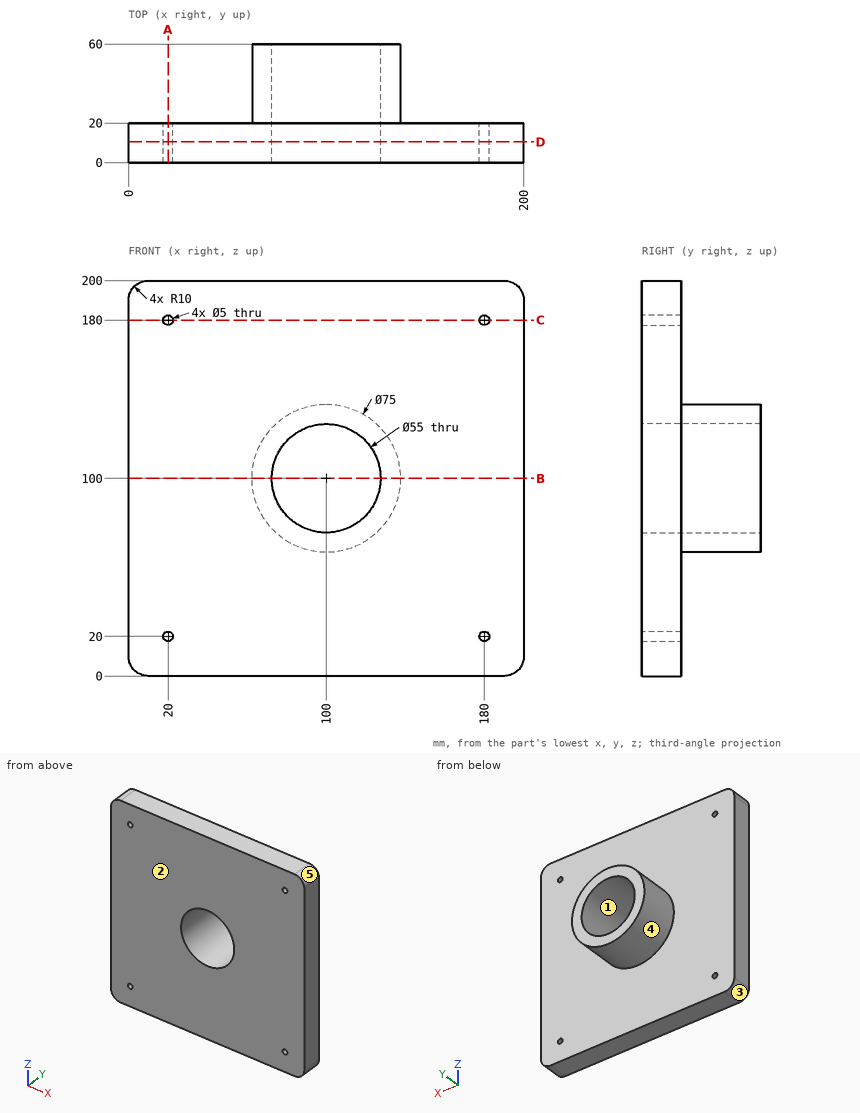
The figure shows three views and two pictorial views of one solid part (mm, origin at its lowest corner). Answer the questions. A direction names the side the tool comes from. Coordinates: 2 decimals unless noted, no trailing zeros. Loops run counter-clockwise (first coordinate to the right, second up) from the corner with the lowest first, then second, coordinate; pieces in that order, holes last. Notation, with made-up numbers: (-35, 66) -> (-5, 66) arc R25 ccw to (-5, 97) -> close; hole circle Ø11 at (-9.5, 19). An arc over 180 degrees is marked (long way). Use one line per item in the form item = value. Start each with the question number.
Item 1: Consider L1, parallel to X at y = 9, z = 180; L2, parallel to Y at x = 101.5, z = 190. Determine where each line is inside the solid, lowest interval first. Write a range as [from, to].
Item 2: Flat-ended cylindrical pins translate along their axes: pin 1 Ø8 at (x, z) = (137, 148) entering from +Y; pin 2 Ø4.5 at (x, z) = (180, 20) entering from +Y. Find the tip coordinate at first contact, or state that the pin passes through.
Item 3: The part is cut by section B-B on z = 100. Determine the outline of the cut face in (x, y), then the cut area to 3 significant figures.
Item 4: The part is cut by section C-C on z = 180. Determine the outline of the cut face in (x, y).
Item 5: The mould has two halves that part along X. Classify the marked faces 1, 2 and 3: released by +X, released by -X, zero draft, split by the parting line, or undercut.
Item 6: The part is cut by section D-D on y = 10.5. Determine the outline of the cut face in (x, z), then the cut area to 3 significant figures.
Item 7: A tool of negligible diameter and unlimited length cuts with its end or side. For the marked faces 4 and 5, from which of +Z, -Z, +X, -X, +Y, -Y can it reach the whole face along a straight path? Write none if from no direction.
Item 8: The part is cut by section A-A on x = 20. Determine the outline of the cut face in (y, z).
Answer key:
q1.L1 = [0, 17.5], [22.5, 177.5], [182.5, 200]
q1.L2 = [0, 20]
q2.pin_1 = 20
q2.pin_2 = through
q3.outline = (0, 0) -> (72.5, 0) -> (72.5, 60) -> (62.5, 60) -> (62.5, 20) -> (0, 20) -> close; (127.5, 0) -> (200, 0) -> (200, 20) -> (137.5, 20) -> (137.5, 60) -> (127.5, 60) -> close
q3.area = 3,700 mm2
q4.outline = (0, 0) -> (17.5, 0) -> (17.5, 20) -> (0, 20) -> close; (22.5, 0) -> (177.5, 0) -> (177.5, 20) -> (22.5, 20) -> close; (182.5, 0) -> (200, 0) -> (200, 20) -> (182.5, 20) -> close
q5.face_1 = undercut
q5.face_2 = zero draft
q5.face_3 = released by -X
q6.outline = (0, 10) arc R10 ccw to (10, 0) -> (190, 0) arc R10 ccw to (200, 10) -> (200, 190) arc R10 ccw to (190, 200) -> (10, 200) arc R10 ccw to (0, 190) -> close; hole circle Ø5 at (20, 20); hole circle Ø5 at (20, 180); hole circle Ø55 at (100, 100); hole circle Ø5 at (180, 20); hole circle Ø5 at (180, 180)
q6.area = 37,500 mm2
q7.face_4 = +Y
q7.face_5 = +Z, +X, +Y, -Y
q8.outline = (0, 0) -> (20, 0) -> (20, 17.5) -> (0, 17.5) -> close; (0, 22.5) -> (20, 22.5) -> (20, 177.5) -> (0, 177.5) -> close; (0, 182.5) -> (20, 182.5) -> (20, 200) -> (0, 200) -> close
